Could you check a few things on this model? Use its own coordinates, in mm. A direction names the side the tool comes from. Coordinates: 2 decimals unless noted, no trailing zeros. Order: outer loops, then holes, each group sorted by start corner. A loop starts at its lowest first (then second) coordinate and runs counter-clockwise, first axis right, second up. Notation, with made-up numbers: (-33, 31.5) - (11, 31.5) arc R23 cw to (11, 59.5) - close; hole circle Ø10 at (10, 70.25). An arc over 180 degrees is marked (long way). One line per item, written item: value.
from build123d import *

# Parameters (mm, degrees)
BOSS_EXTRUDE1_DEPTH      = 10
BOSS_EXTRUDE1_DEPTH_BACK = 74
SKETCH3_W                = 64
SKETCH3_H                = 550
CUT_EXTRUDE1_DEPTH       = 890
SKETCH4_W                = 64
SKETCH4_H                = 350
BOSS_EXTRUDE2_DEPTH      = 10
SKETCH5_W                = 64
SKETCH5_H                = 190
BOSS_EXTRUDE3_DEPTH      = 10
CUT_EXTRUDE2_REACH       = 712
SKETCH6_R                = 4.5
CUT_EXTRUDE3_REACH       = 76
SKETCH7_R                = 8
CUT_EXTRUDE4_REACH       = 12
SKETCH8_R                = 4.5
SKETCH8_R_2              = 5


with BuildPart() as part:
    # Sketch1 → Boss-Extrude1 (new body, two sides)
    with BuildSketch(Plane(origin=(0, 0, 0), x_dir=(0, 0, -1), z_dir=(1, 0, 0))) as boss_extrude1_sk:
        Polygon((0, 0), (0, 750), (150, 900), (550, 900), (550, 700), (200, 700), (200, 0), align=None)
    extrude(amount=BOSS_EXTRUDE1_DEPTH)
    extrude(boss_extrude1_sk.sketch, amount=-BOSS_EXTRUDE1_DEPTH_BACK)

    # Sketch3 → Cut-Extrude1 (cut)
    with BuildSketch(Plane(origin=(0, 900, 0), x_dir=(1, 0, 0), z_dir=(0, 1, 0))):
        with Locations((-32, 275)):
            Rectangle(SKETCH3_W, SKETCH3_H)
    extrude(amount=-CUT_EXTRUDE1_DEPTH, mode=Mode.SUBTRACT)

    # Sketch4 → Boss-Extrude2 (add)
    with BuildSketch(Plane.XZ.offset(-700)):
        with Locations((-32, -375)):
            Rectangle(SKETCH4_W, SKETCH4_H)
    extrude(amount=-BOSS_EXTRUDE2_DEPTH)

    # Sketch5 → Boss-Extrude3 (add)
    with BuildSketch(Plane(origin=(0, 0, -486), x_dir=(-1, 0, 0), z_dir=(0, 0, -1))):
        with Locations((32, 805)):
            Rectangle(SKETCH5_W, SKETCH5_H)
    extrude(amount=-BOSS_EXTRUDE3_DEPTH)

    # Sketch6 → Cut-Extrude2 (cut, up to next)
    with BuildSketch(Plane(origin=(0, 710, 0), x_dir=(1, 0, 0), z_dir=(0, 1, 0)), mode=Mode.PRIVATE) as cut_extrude2_sk1:
        with Locations((-8.5, 494.5)):
            Circle(SKETCH6_R)
    cut_extrude2_tool1 = extrude(cut_extrude2_sk1.sketch, amount=-CUT_EXTRUDE2_REACH, mode=Mode.PRIVATE) & part.part
    add(cut_extrude2_tool1.solids().sort_by_distance((-8.5, 710, -494.5))[0], mode=Mode.SUBTRACT)
    # Sketch6 → Cut-Extrude2 (cut, up to next)
    with BuildSketch(Plane(origin=(0, 710, 0), x_dir=(1, 0, 0), z_dir=(0, 1, 0)), mode=Mode.PRIVATE) as cut_extrude2_sk2:
        with Locations((-55, 494.5)):
            Circle(SKETCH6_R)
    cut_extrude2_tool2 = extrude(cut_extrude2_sk2.sketch, amount=-CUT_EXTRUDE2_REACH, mode=Mode.PRIVATE) & part.part
    add(cut_extrude2_tool2.solids().sort_by_distance((-55, 710, -494.5))[0], mode=Mode.SUBTRACT)
    # Sketch6 → Cut-Extrude2 (cut, up to next)
    with BuildSketch(Plane(origin=(0, 710, 0), x_dir=(1, 0, 0), z_dir=(0, 1, 0)), mode=Mode.PRIVATE) as cut_extrude2_sk3:
        with Locations((-55, 541)):
            Circle(SKETCH6_R)
    cut_extrude2_tool3 = extrude(cut_extrude2_sk3.sketch, amount=-CUT_EXTRUDE2_REACH, mode=Mode.PRIVATE) & part.part
    add(cut_extrude2_tool3.solids().sort_by_distance((-55, 710, -541))[0], mode=Mode.SUBTRACT)
    # Sketch6 → Cut-Extrude2 (cut, up to next)
    with BuildSketch(Plane(origin=(0, 710, 0), x_dir=(1, 0, 0), z_dir=(0, 1, 0)), mode=Mode.PRIVATE) as cut_extrude2_sk4:
        with Locations((-8.5, 541)):
            Circle(SKETCH6_R)
    cut_extrude2_tool4 = extrude(cut_extrude2_sk4.sketch, amount=-CUT_EXTRUDE2_REACH, mode=Mode.PRIVATE) & part.part
    add(cut_extrude2_tool4.solids().sort_by_distance((-8.5, 710, -541))[0], mode=Mode.SUBTRACT)

    # Sketch7 → Cut-Extrude3 (cut, up to next)
    with BuildSketch(Plane.XY.offset(-476), mode=Mode.PRIVATE) as cut_extrude3_sk1:
        with Locations((-26.25, 732.5)):
            Circle(SKETCH7_R)
    cut_extrude3_tool1 = extrude(cut_extrude3_sk1.sketch, amount=-CUT_EXTRUDE3_REACH, mode=Mode.PRIVATE) & part.part
    add(cut_extrude3_tool1.solids().sort_by_distance((-26.25, 732.5, -476))[0], mode=Mode.SUBTRACT)

    # Sketch8 → Cut-Extrude4 (cut, up to next)
    with BuildSketch(Plane(origin=(0, 10, 0), x_dir=(1, 0, 0), z_dir=(0, 1, 0)), mode=Mode.PRIVATE) as cut_extrude4_sk1:
        with Locations((-54.5, 185)):
            Circle(SKETCH8_R)
    cut_extrude4_tool1 = extrude(cut_extrude4_sk1.sketch, amount=-CUT_EXTRUDE4_REACH, mode=Mode.PRIVATE) & part.part
    add(cut_extrude4_tool1.solids().sort_by_distance((-54.5, 10, -185))[0], mode=Mode.SUBTRACT)
    # Sketch8 → Cut-Extrude4 (cut, up to next)
    with BuildSketch(Plane(origin=(0, 10, 0), x_dir=(1, 0, 0), z_dir=(0, 1, 0)), mode=Mode.PRIVATE) as cut_extrude4_sk2:
        with Locations((-54.5, 165)):
            Circle(SKETCH8_R_2)
    cut_extrude4_tool2 = extrude(cut_extrude4_sk2.sketch, amount=-CUT_EXTRUDE4_REACH, mode=Mode.PRIVATE) & part.part
    add(cut_extrude4_tool2.solids().sort_by_distance((-54.5, 10, -165))[0], mode=Mode.SUBTRACT)
    # Sketch8 → Cut-Extrude4 (cut, up to next)
    with BuildSketch(Plane(origin=(0, 10, 0), x_dir=(1, 0, 0), z_dir=(0, 1, 0)), mode=Mode.PRIVATE) as cut_extrude4_sk3:
        with Locations((-54.5, 15)):
            Circle(SKETCH8_R)
    cut_extrude4_tool3 = extrude(cut_extrude4_sk3.sketch, amount=-CUT_EXTRUDE4_REACH, mode=Mode.PRIVATE) & part.part
    add(cut_extrude4_tool3.solids().sort_by_distance((-54.5, 10, -15))[0], mode=Mode.SUBTRACT)
    # Sketch8 → Cut-Extrude4 (cut, up to next)
    with BuildSketch(Plane(origin=(0, 10, 0), x_dir=(1, 0, 0), z_dir=(0, 1, 0)), mode=Mode.PRIVATE) as cut_extrude4_sk4:
        with Locations((-9.5, 15)):
            Circle(SKETCH8_R)
    cut_extrude4_tool4 = extrude(cut_extrude4_sk4.sketch, amount=-CUT_EXTRUDE4_REACH, mode=Mode.PRIVATE) & part.part
    add(cut_extrude4_tool4.solids().sort_by_distance((-9.5, 10, -15))[0], mode=Mode.SUBTRACT)
    # Sketch8 → Cut-Extrude4 (cut, up to next)
    with BuildSketch(Plane(origin=(0, 10, 0), x_dir=(1, 0, 0), z_dir=(0, 1, 0)), mode=Mode.PRIVATE) as cut_extrude4_sk5:
        with Locations((-9.5, 35)):
            Circle(SKETCH8_R_2)
    cut_extrude4_tool5 = extrude(cut_extrude4_sk5.sketch, amount=-CUT_EXTRUDE4_REACH, mode=Mode.PRIVATE) & part.part
    add(cut_extrude4_tool5.solids().sort_by_distance((-9.5, 10, -35))[0], mode=Mode.SUBTRACT)
    # Sketch8 → Cut-Extrude4 (cut, up to next)
    with BuildSketch(Plane(origin=(0, 10, 0), x_dir=(1, 0, 0), z_dir=(0, 1, 0)), mode=Mode.PRIVATE) as cut_extrude4_sk6:
        with Locations((-9.5, 185)):
            Circle(SKETCH8_R)
    cut_extrude4_tool6 = extrude(cut_extrude4_sk6.sketch, amount=-CUT_EXTRUDE4_REACH, mode=Mode.PRIVATE) & part.part
    add(cut_extrude4_tool6.solids().sort_by_distance((-9.5, 10, -185))[0], mode=Mode.SUBTRACT)


solid = part.part
Item 1: I'm going to push flat-ended pins straight in: pin 1 Ø5 at (x, y) = (0.5, 362.5) entering from +Z; pin 2 Ø7 at (x, z) = (-54.5, -15) entering from +Y; pin 3 Ø5 at (x, z) = (-9.5, -348.5) entering from +Y; pin 4 Ø12 at (x, z) = (-46, -129.5) entering from +Y. Where does each tip first touch, or does it pass through?
Conclusion:
pin 1: z = 0
pin 2: through
pin 3: y = 710
pin 4: y = 10
Item 2: I want a section at C-C on z = -423. Please give me the cut outline in (x, y).
Conclusion:
outline: (-74, 700) - (10, 700) - (10, 900) - (0, 900) - (0, 710) - (-64, 710) - (-64, 900) - (-74, 900) - close
Item 3: I want a section at A-A on z = -80. Please give me the cut outline in (x, y), then the cut area to 3 significant figures.
Conclusion:
outline: (-74, 0) - (10, 0) - (10, 830) - (0, 830) - (0, 10) - (-64, 10) - (-64, 830) - (-74, 830) - close
area: 17,200 mm²
Item 4: I want a section at B-B on y = 475.5. Please give me the cut outline in (x, z), then the cut area to 3 significant figures.
Conclusion:
outline: (-74, -200) - (-64, -200) - (-64, 0) - (-74, 0) - close; (0, -200) - (10, -200) - (10, 0) - (0, 0) - close
area: 4,000 mm²
Item 5: For faces 5 (the face through (-33, 700, -373)), 6 (the face through (5, 824, -74)), 7 (the face through (0, 560, -182)), 8 (the face through (0, 806, -518)), 9 (the face through (-22.56, 725.4, -480.93)), which set-ups out of +Z, -Z, +X, -X, +Y, -Y let a thin tool reach every point of the face, with its end or its side?
Conclusion:
face 5: -Z, +X, -X, -Y
face 6: +Z, +X, -X, +Y
face 7: +Z, +Y
face 8: -Z, +Y
face 9: +Z, -Z
Item 6: Thinking about a two-plate mould opening in X: for faces 1 (the face through (10, 556, -157)), 2 (the face through (-31, 0, -101)), 3 (the face through (-32, 10, -101)), 4 (the face through (-32, 806, -476)), which applies, pulls with the +X half, pulls with the -X half, needs draft (parallel to the pull), parting line crosses it, or undercut?
Conclusion:
face 1: pulls with the +X half
face 2: needs draft
face 3: undercut
face 4: undercut
Item 7: If I drill on probe 1 along X at (y, z) = (706.75, -541); probe 2 along Z at (x, y) = (-8, 706); probe 3 along X at (y, z) = (6.5, -15), over which ranges is the centre line in solid material (lowest first)?
Conclusion:
probe 1: -74 to -59.5, -50.5 to -13, -4 to 10
probe 2: -550 to -545.47, -536.53 to -498.97, -490.03 to -200
probe 3: -74 to -59, -50 to -14, -5 to 10
